Input: part model. Units: mm. Frame: model coordinates. Face numbers are marked on the shaded views. A direction names the side the tool comes from. Coordinates: 2 decimals unless noted, no trailing zeros. Write each loop counter-clockwise with the first axis right and the second up, starting at its lowest first coordinate (ties: lowest second). Pieces come first, ordered by that corner, then holes. Notation, with made-up numbers: M 60,-31.75 L 69,-31.75 A9 ccw 69,-23.75 Z; hole C -38.5,30.5 d3. An arc over 180 degrees is marked long. Write each question's results on one line, items separated by ' | '. Start each with the question number.
1. Section query A-A, the plane y = 0. Output: boundary loops of the cut face in (x, z), and give its area (3 significant figures).
2. Section query B-B, the plane x = 20. Output: boundary loops of the cut face in (y, z), and give its area (3 significant figures).
3. Ray query, probe 1 along Y at (x, z) = (0, -9.4); probe 2 along X at (y, z) = (29.5, -11); probe 3 along Z at (x, y) = (-1, -34.5). Return the intervals inside material, ascending.
4. Set-up query: the marked faces 1 and 2. Return all of +Z, -Z, +X, -X, +Y, -Y with unobstructed straight access to the full face (end or side cutting, diameter ignored); none if empty.
5. Section query C-C, the plane z = -10. Count the separate pieces of the cut face and the enclosed holes in it, and give its area (3 significant figures).
6. First-contact query: pin 1 (2.5 mm diameter, centred on x = -2, y = 30, fed in from +Z); pin 2 (3 mm diameter, centred on x = -6.5, z = 3, fed in from +Y); pin 3 (8.5 mm diameter, centred on x = -54, y = 0, fed in from +Z). Flat tips, straight axial feed; report the tip coordinate or a pass-through.
7. Section query D-D, the plane y = 45. Output: boundary loops of the cut face in (x, z), and give its area (3 significant figures).
```python
from build123d import *

# Parameters (mm, degrees)
F_01_START                                     = -12
S01_ROUNDED_V3_BACKPLATE_WITH_CAGE_AND_R       = 3.3
S01_ROUNDED_V3_BACKPLATE_WITH_CAGE_AND_R_2     = 2.25
F_01_ROUNDED_V3_BACKPLATE_WITH_CAGE_AND_DEPTH  = 6
F_02_START                                     = -6
S02_THREE_CORD_GUIDE_PEDESTALS_R               = 4.35
F_02_THREE_CORD_GUIDE_PEDESTALS_DEPTH          = 5
F_03_START                                     = -13
S03_THREE_SMOOTH_GROMMET_SEATS_R               = 2.05
F_03_THREE_SMOOTH_GROMMET_SEATS_DEPTH          = 14
F_04_START                                     = -7.2
F_04_INTEGRAL_A1_FORK_CHEEK_L_DEPTH            = 3.6
F_05_START                                     = 3.6
F_05_INTEGRAL_A1_FORK_CHEEK_R_DEPTH            = 3.6
F_06_START                                     = -7.5
S06_A1_PIVOT_THROUGH_BOTH_CHEEKS_R             = 1.65
F_06_A1_PIVOT_THROUGH_BOTH_CHEEKS_DEPTH        = 15
F_07_START                                     = -7.3
S07_A1_RECESSED_PIVOT_SCREW_HEAD_R             = 2.7
F_07_A1_RECESSED_PIVOT_SCREW_HEAD_DEPTH        = 1.5
F_08_START                                     = -7.2
F_08_INTEGRAL_A2_FORK_CHEEK_L_DEPTH            = 3.6
F_09_START                                     = 3.6
F_09_INTEGRAL_A2_FORK_CHEEK_R_DEPTH            = 3.6
F_10_START                                     = -7.5
S10_A2_PIVOT_THROUGH_BOTH_CHEEKS_R             = 1.65
F_10_A2_PIVOT_THROUGH_BOTH_CHEEKS_DEPTH        = 15
F_11_START                                     = -7.3
S11_A2_RECESSED_PIVOT_SCREW_HEAD_R             = 2.7
F_11_A2_RECESSED_PIVOT_SCREW_HEAD_DEPTH        = 1.5
F_12_START                                     = -7.2
F_12_INTEGRAL_A3_FORK_CHEEK_L_DEPTH            = 3.6
F_13_START                                     = 3.6
F_13_INTEGRAL_A3_FORK_CHEEK_R_DEPTH            = 3.6
F_14_START                                     = -7.5
S14_A3_PIVOT_THROUGH_BOTH_CHEEKS_R             = 1.65
F_14_A3_PIVOT_THROUGH_BOTH_CHEEKS_DEPTH        = 15
F_15_START                                     = -7.3
S15_A3_RECESSED_PIVOT_SCREW_HEAD_R             = 2.7
F_15_A3_RECESSED_PIVOT_SCREW_HEAD_DEPTH        = 1.5
F_16_START                                     = -12
F_16_CONTINUOUS_LAND_FOR_BUMP_END_SUPPOR_DEPTH = 6
F_17_START                                     = -12.1
S17_THROUGH_CLEARANCE_FOR_TRACK_SUPPOR_R       = 3.3
F_17_THROUGH_CLEARANCE_FOR_TRACK_SUPPORT_DEPTH = 6.2
F_18_START                                     = -8.5
S18_LOCATING_COUNTERBORE_FOR_BUMP_END_R        = 5.1
F_18_LOCATING_COUNTERBORE_FOR_BUMP_END_P_DEPTH = 2.6


with BuildPart() as part:
    # S01 - Rounded V3 backplate with cage and cassette fixings → 01 - Rounded V3 backplate with cage and cassette fixings (new body)
    with BuildSketch(Plane.XY.offset(F_01_START)):
        with BuildLine():
            Line((-61.28, -5.46), (-22.28, -57.46))
            ThreePointArc((-22.28, -57.46), (-19.599751768, -59.85189682), (-16.202689853, -61.020173896))
            Line((-16.202689853, -61.020173896), (-1.202689853, -63.020173896))
            ThreePointArc((-1.202689853, -63.020173896), (3.754538811, -62.28935693), (7.573381448, -59.045185174))
            Line((7.573381448, -59.045185174), (33.554143562, -20.045185174))
            ThreePointArc((33.554143562, -20.045185174), (34.27222658, -18.749882266), (34.770687133, -17.35525331))
            Line((34.770687133, -17.35525331), (38.789925019, -2.35525331))
            ThreePointArc((38.789925019, -2.35525331), (39.031640499, 1.113314824), (37.954831213, 4.419350674))
            Line((37.954831213, 4.419350674), (7.954831213, 58.419350674))
            ThreePointArc((7.954831213, 58.419350674), (0.151603518, 63.098737076), (-7.803185624, 58.681911374))
            Line((-7.803185624, 58.681911374), (-29.111780005, 23.167587405))
            ThreePointArc((-29.111780005, 23.167587405), (-30.615922322, 21.34087773), (-32.588639688, 20.034088329))
            Line((-32.588639688, 20.034088329), (-57.848257735, 8.246266574))
            ThreePointArc((-57.848257735, 8.246266574), (-62.827511875, 2.210211325), (-61.28, -5.46))
        make_face()
        with Locations((0, 54)):
            Circle(S01_ROUNDED_V3_BACKPLATE_WITH_CAGE_AND_R, mode=Mode.SUBTRACT)
        with Locations((-54, 0)):
            Circle(S01_ROUNDED_V3_BACKPLATE_WITH_CAGE_AND_R, mode=Mode.SUBTRACT)
        with Locations((0, -54)):
            Circle(S01_ROUNDED_V3_BACKPLATE_WITH_CAGE_AND_R, mode=Mode.SUBTRACT)
        with Locations((14, -12)):
            Circle(S01_ROUNDED_V3_BACKPLATE_WITH_CAGE_AND_R_2, mode=Mode.SUBTRACT)
        with Locations((20, 14)):
            Circle(S01_ROUNDED_V3_BACKPLATE_WITH_CAGE_AND_R_2, mode=Mode.SUBTRACT)
        with Locations((-24, 0)):
            Circle(S01_ROUNDED_V3_BACKPLATE_WITH_CAGE_AND_R_2, mode=Mode.SUBTRACT)
    extrude(amount=F_01_ROUNDED_V3_BACKPLATE_WITH_CAGE_AND_DEPTH)

    # S02 - Three cord guide pedestals → 02 - Three cord guide pedestals (add)
    with BuildSketch(Plane.XY.offset(F_02_START)):
        with Locations((25.980762114, -15)):
            Circle(S02_THREE_CORD_GUIDE_PEDESTALS_R)
        with Locations((0, 30)):
            Circle(S02_THREE_CORD_GUIDE_PEDESTALS_R)
        with Locations((-25.980762114, -15)):
            Circle(S02_THREE_CORD_GUIDE_PEDESTALS_R)
    extrude(amount=F_02_THREE_CORD_GUIDE_PEDESTALS_DEPTH)

    # S03 - Three smooth grommet seats → 03 - Three smooth grommet seats (cut)
    with BuildSketch(Plane.XY.offset(F_03_START)):
        with Locations((25.980762114, -15)):
            Circle(S03_THREE_SMOOTH_GROMMET_SEATS_R)
        with Locations((0, 30)):
            Circle(S03_THREE_SMOOTH_GROMMET_SEATS_R)
        with Locations((-25.980762114, -15)):
            Circle(S03_THREE_SMOOTH_GROMMET_SEATS_R)
    extrude(amount=F_03_THREE_SMOOTH_GROMMET_SEATS_DEPTH, mode=Mode.SUBTRACT)

    # S04 - Integral A1 fork cheek L → 04 - Integral A1 fork cheek L (add)
    with BuildSketch(Plane(origin=(2.009618943, -7.5, 0), x_dir=(0.9659258262890683, 0.25881904510252085, 0), z_dir=(-0.2588190451025208, 0.9659258262890682, 0)).offset(F_04_START)):
        with BuildLine():
            Line((35.077774789, 7), (22.877774789, 7))
            Line((22.877774789, 7), (24.027774789, 0))
            ThreePointArc((24.027774789, 0), (28.977774789, -4.95), (33.927774789, 0))
            Line((33.927774789, 0), (35.077774789, 7))
        make_face()
    extrude(amount=F_04_INTEGRAL_A1_FORK_CHEEK_L_DEPTH)

    # S05 - Integral A1 fork cheek R → 05 - Integral A1 fork cheek R (add)
    with BuildSketch(Plane(origin=(2.009618943, -7.5, 0), x_dir=(0.9659258262890683, 0.25881904510252085, 0), z_dir=(-0.2588190451025208, 0.9659258262890682, 0)).offset(F_05_START)):
        with BuildLine():
            Line((35.077774789, 7), (22.877774789, 7))
            Line((22.877774789, 7), (24.027774789, 0))
            ThreePointArc((24.027774789, 0), (28.977774789, -4.95), (33.927774789, 0))
            Line((33.927774789, 0), (35.077774789, 7))
        make_face()
    extrude(amount=F_05_INTEGRAL_A1_FORK_CHEEK_R_DEPTH)

    # S06 - A1 pivot through both cheeks → 06 - A1 pivot through both cheeks (cut)
    with BuildSketch(Plane(origin=(2.009618943, -7.5, 0), x_dir=(0.9659258262890683, 0.25881904510252085, 0), z_dir=(-0.2588190451025208, 0.9659258262890682, 0)).offset(F_06_START)):
        with Locations((28.977774789, 0)):
            Circle(S06_A1_PIVOT_THROUGH_BOTH_CHEEKS_R)
    extrude(amount=F_06_A1_PIVOT_THROUGH_BOTH_CHEEKS_DEPTH, mode=Mode.SUBTRACT)

    # S07 - A1 recessed pivot screw head → 07 - A1 recessed pivot screw head (cut)
    with BuildSketch(Plane(origin=(2.009618943, -7.5, 0), x_dir=(0.9659258262890683, 0.25881904510252085, 0), z_dir=(-0.2588190451025208, 0.9659258262890682, 0)).offset(F_07_START)):
        with Locations(Location((28.977774789, 0, 0), (0, 0, 180))):
            Circle(S07_A1_RECESSED_PIVOT_SCREW_HEAD_R)
    extrude(amount=F_07_A1_RECESSED_PIVOT_SCREW_HEAD_DEPTH, mode=Mode.SUBTRACT)

    # S08 - Integral A2 fork cheek L → 08 - Integral A2 fork cheek L (add)
    with BuildSketch(Plane(origin=(5.490381057, 5.490381057, 0), x_dir=(-0.7071067811865475, 0.7071067811865477, 0), z_dir=(-0.7071067811865477, -0.7071067811865475, 0)).offset(F_08_START)):
        with BuildLine():
            Line((35.077774789, 7), (22.877774789, 7))
            Line((22.877774789, 7), (24.027774789, 0))
            ThreePointArc((24.027774789, 0), (28.977774789, -4.95), (33.927774789, 0))
            Line((33.927774789, 0), (35.077774789, 7))
        make_face()
    extrude(amount=F_08_INTEGRAL_A2_FORK_CHEEK_L_DEPTH)

    # S09 - Integral A2 fork cheek R → 09 - Integral A2 fork cheek R (add)
    with BuildSketch(Plane(origin=(5.490381057, 5.490381057, 0), x_dir=(-0.7071067811865475, 0.7071067811865477, 0), z_dir=(-0.7071067811865477, -0.7071067811865475, 0)).offset(F_09_START)):
        with BuildLine():
            Line((35.077774789, 7), (22.877774789, 7))
            Line((22.877774789, 7), (24.027774789, 0))
            ThreePointArc((24.027774789, 0), (28.977774789, -4.95), (33.927774789, 0))
            Line((33.927774789, 0), (35.077774789, 7))
        make_face()
    extrude(amount=F_09_INTEGRAL_A2_FORK_CHEEK_R_DEPTH)

    # S10 - A2 pivot through both cheeks → 10 - A2 pivot through both cheeks (cut)
    with BuildSketch(Plane(origin=(5.490381057, 5.490381057, 0), x_dir=(-0.7071067811865475, 0.7071067811865477, 0), z_dir=(-0.7071067811865477, -0.7071067811865475, 0)).offset(F_10_START)):
        with Locations(Location((28.977774789, 0, 0), (0, 0, 180))):
            Circle(S10_A2_PIVOT_THROUGH_BOTH_CHEEKS_R)
    extrude(amount=F_10_A2_PIVOT_THROUGH_BOTH_CHEEKS_DEPTH, mode=Mode.SUBTRACT)

    # S11 - A2 recessed pivot screw head → 11 - A2 recessed pivot screw head (cut)
    with BuildSketch(Plane(origin=(5.490381057, 5.490381057, 0), x_dir=(-0.7071067811865475, 0.7071067811865477, 0), z_dir=(-0.7071067811865477, -0.7071067811865475, 0)).offset(F_11_START)):
        with Locations(Location((28.977774789, 0, 0), (0, 0, 180))):
            Circle(S11_A2_RECESSED_PIVOT_SCREW_HEAD_R)
    extrude(amount=F_11_A2_RECESSED_PIVOT_SCREW_HEAD_DEPTH, mode=Mode.SUBTRACT)

    # S12 - Integral A3 fork cheek L → 12 - Integral A3 fork cheek L (add)
    with BuildSketch(Plane(origin=(-7.5, 2.009618943, 0), x_dir=(0, 0, -1), z_dir=(0.9659258262890683, -0.25881904510252113, 0)).offset(F_12_START)):
        with BuildLine():
            Line((7, -35.077774789), (7, -22.877774789))
            Line((7, -22.877774789), (0, -24.027774789))
            ThreePointArc((0, -24.027774789), (-4.95, -28.977774789), (0, -33.927774789))
            Line((0, -33.927774789), (7, -35.077774789))
        make_face()
    extrude(amount=F_12_INTEGRAL_A3_FORK_CHEEK_L_DEPTH)

    # S13 - Integral A3 fork cheek R → 13 - Integral A3 fork cheek R (add)
    with BuildSketch(Plane(origin=(-7.5, 2.009618943, 0), x_dir=(0, 0, -1), z_dir=(0.9659258262890683, -0.25881904510252113, 0)).offset(F_13_START)):
        with BuildLine():
            Line((7, -35.077774789), (7, -22.877774789))
            Line((7, -22.877774789), (0, -24.027774789))
            ThreePointArc((0, -24.027774789), (-4.95, -28.977774789), (0, -33.927774789))
            Line((0, -33.927774789), (7, -35.077774789))
        make_face()
    extrude(amount=F_13_INTEGRAL_A3_FORK_CHEEK_R_DEPTH)

    # S14 - A3 pivot through both cheeks → 14 - A3 pivot through both cheeks (cut)
    with BuildSketch(Plane(origin=(-7.5, 2.009618943, 0), x_dir=(0, 0, -1), z_dir=(0.9659258262890683, -0.25881904510252113, 0)).offset(F_14_START)):
        with Locations(Location((0, -28.977774789, 0), (0, 0, 90))):
            Circle(S14_A3_PIVOT_THROUGH_BOTH_CHEEKS_R)
    extrude(amount=F_14_A3_PIVOT_THROUGH_BOTH_CHEEKS_DEPTH, mode=Mode.SUBTRACT)

    # S15 - A3 recessed pivot screw head → 15 - A3 recessed pivot screw head (cut)
    with BuildSketch(Plane(origin=(-7.5, 2.009618943, 0), x_dir=(0, 0, -1), z_dir=(0.9659258262890683, -0.25881904510252113, 0)).offset(F_15_START)):
        with Locations(Location((0, -28.977774789, 0), (0, 0, 90))):
            Circle(S15_A3_RECESSED_PIVOT_SCREW_HEAD_R)
    extrude(amount=F_15_A3_RECESSED_PIVOT_SCREW_HEAD_DEPTH, mode=Mode.SUBTRACT)

    # S16 - Continuous land for bump end support → 16 - Continuous land for bump end support (add)
    with BuildSketch(Plane.XY.offset(F_16_START)):
        with BuildLine():
            Line((18.50606906, 7.339296649), (42.793274403, 38.756619219))
            ThreePointArc((42.793274403, 38.756619219), (59.626501992, 40.91125351), (61.781136283, 24.07802592))
            Line((61.781136283, 24.07802592), (37.49393094, -7.339296649))
            ThreePointArc((37.49393094, -7.339296649), (20.660703351, -9.49393094), (18.50606906, 7.339296649))
        make_face()
    extrude(amount=F_16_CONTINUOUS_LAND_FOR_BUMP_END_SUPPOR_DEPTH)

    # S17 - Through clearance for track support screw → 17 - Through clearance for track support screw (cut)
    with BuildSketch(Plane.XY.offset(F_17_START)):
        with Locations((52.287205343, 31.41732257)):
            Circle(S17_THROUGH_CLEARANCE_FOR_TRACK_SUPPOR_R)
    extrude(amount=F_17_THROUGH_CLEARANCE_FOR_TRACK_SUPPORT_DEPTH, mode=Mode.SUBTRACT)

    # S18 - Locating counterbore for bump end post → 18 - Locating counterbore for bump end post (cut)
    with BuildSketch(Plane.XY.offset(F_18_START)):
        with Locations((52.287205343, 31.41732257)):
            Circle(S18_LOCATING_COUNTERBORE_FOR_BUMP_END_R)
    extrude(amount=F_18_LOCATING_COUNTERBORE_FOR_BUMP_END_P_DEPTH, mode=Mode.SUBTRACT)


solid = part.part
```
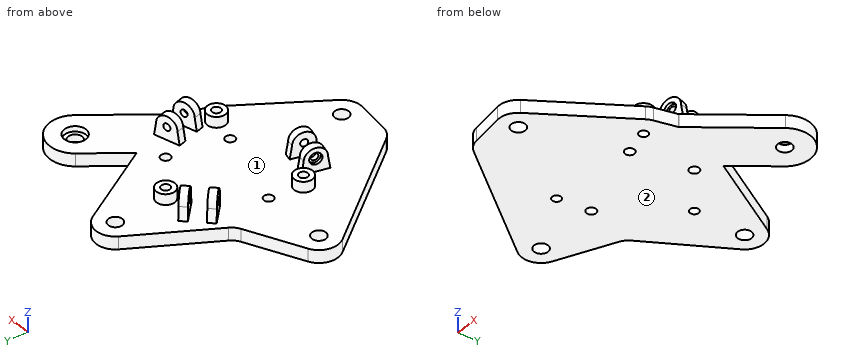
Answer:
1) outline: M -63.1,-12 L -57.3,-12 L -57.3,-6 L -63.1,-6 Z; M -50.7,-12 L -26.25,-12 L -26.25,-6 L -50.7,-6 Z; M -21.75,-12 L 43.17,-12 L 43.17,-6 L -21.75,-6 Z | area: 571 mm^2
2) outline: M -40.39,-12 L 11.75,-12 L 11.75,-6 L -40.39,-6 Z; M 16.25,-12 L 36.74,-12 L 36.74,-6 L 16.25,-6 Z | area: 436 mm^2
3) probe 1: -63.1 to -57.3, -50.7 to 27.95, 32.05 to 50.7, 57.3 to 63.1 | probe 2: -25.31 to -1.99, 1.99 to 24.02, 35.64 to 49.6, 54.97 to 64.13 | probe 3: -12 to -6
4) face 1: +Z | face 2: -Z, +X, -X, +Y, -Y
5) separate pieces: 1 | enclosed holes: 10 | area: 8,100 mm^2
6) pin 1: z = -1 | pin 2: y = 29.16 | pin 3: z = -6
7) outline: M -16.01,-12 L 15.41,-12 L 15.41,-6 L -16.01,-6 Z | area: 189 mm^2
